Here's the drawing with two shaded views (mm, measured from the low corner). I have some questions. A direction names the side the tool comes from. Coordinates: 2 decimals unless noted, no trailing zeros. Write each loop counter-clockwise with the first axis right and the second up, starting at its lowest first coordinate (ties: lowest second). Pieces come first, ordered by that corner, then holes.
Item 1: If I drill on probe 1 along X at (y, z) = (5.5, 7); probe 2 along X at (y, z) = (0.5, 2.75); probe 3 along Z at (x, y) = (7.5, 3) (1 decimal), over which ranges is the centre line in solid material (lowest first)?
Item 2: I want a section at B-B on y = 4.5. Please give me the cut outline in (x, z).
Item 3: Which directions (+Z, -Z, +X, -X, +Y, -Y) give clear straight access to the entire face, cutting with the end or side of a thin tool? Please do the marked faces 4, 5, 6 and 7.
Item 4: I want a section at A-A on x = 3.75. Please give me the cut outline in (y, z).
Item 5: For P1, Ø3, axis at x = 2, z = 3.5, coming from the -Y side; P2, Ø1.6, axis at x = 8, z = 0.5, coming from the +Y side (1 decimal); P3, Ø1, axis at x = 1, y = 3, coming from the -Z side, each with a flat end and sliding along its axis, tell me the tip position at first contact or that it passes through.
Item 6: Thinking about a two-plate mould opening in Z: for the marked faces 1, 2 and 3, which applies, +Z half, -Z half, draft (parallel to the pull), parting line (faces both ways), or undercut?
Item 7: I want a section at D-D on x = 5.25. Please give me the cut outline in (y, z).
Item 8: I want a section at C-C on z = 7. Please give me the cut outline in (x, y).
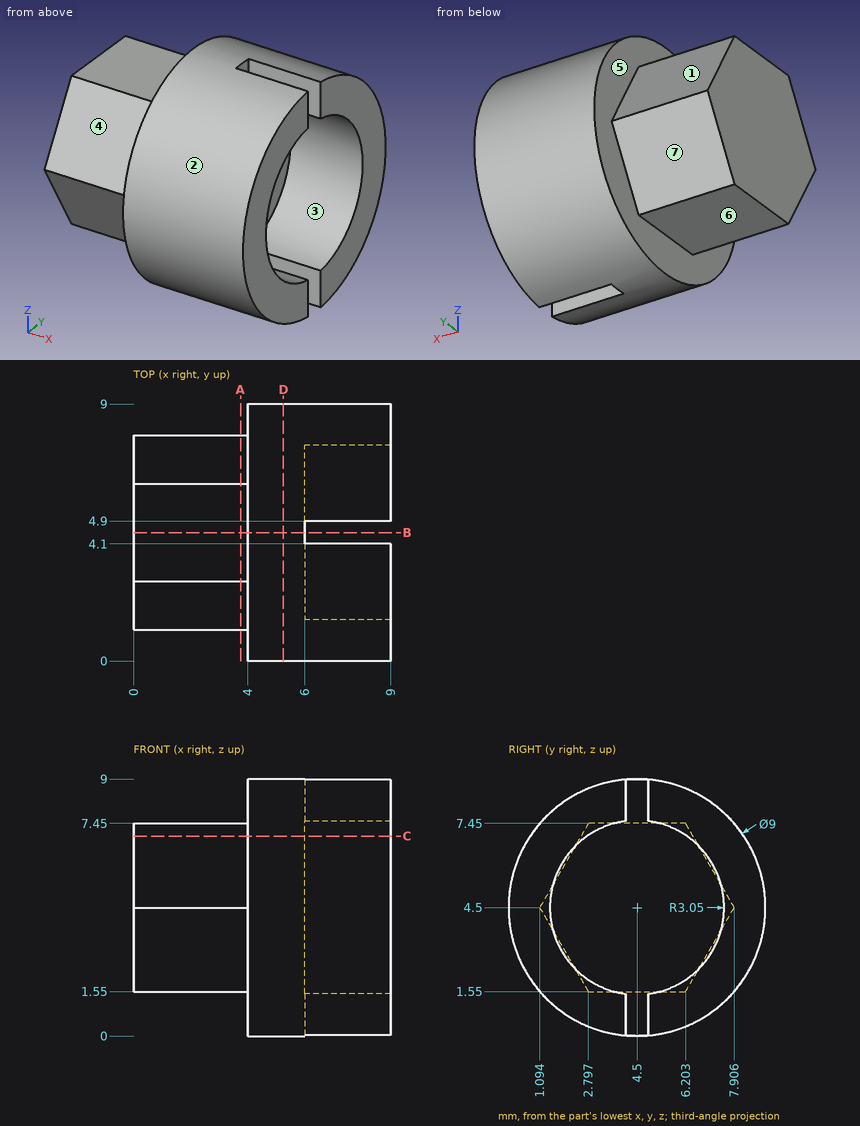
Response values:
1. probe 1: x = 0 to 6
1. probe 2: x = 4 to 9
1. probe 3: z = 0.3 to 1.8, 7.2 to 8.7
2. outline: (0, 1.55) - (4, 1.55) - (4, 0) - (6, 0) - (6, 9) - (4, 9) - (4, 7.45) - (0, 7.45) - close
3. face 4: +Z, -X, -Y
3. face 5: -X
3. face 6: -Z, -X, +Y, -Y
3. face 7: -Z, -X, +Y
4. outline: (1.09, 4.5) - (2.8, 1.55) - (6.2, 1.55) - (7.91, 4.5) - (6.2, 7.45) - (2.8, 7.45) - close
5. P1: stops at y = 1.09
5. P2: stops at y = 7.7
5. P3: stops at z = 1.55
6. face 1: +Z half
6. face 2: parting line
6. face 3: undercut
7. outline: circle Ø9 at (4.5, 4.5)
8. outline: (0, 2.54) - (4, 2.54) - (4, 0.76) - (9, 0.76) - (9, 2.75) - (6, 2.75) - (6, 6.25) - (9, 6.25) - (9, 8.24) - (4, 8.24) - (4, 6.46) - (0, 6.46) - close
